from build123d import *

# Parameters (mm, degrees)
F0_R     = 2
F1_DEPTH = 12
F2_SIZE  = 2.286
F3_SIZE  = 2.286
F4_R     = 2.08915
F5_DEPTH = 219.3935


with BuildPart() as f1:
    # F0 (on Top) → F1 (new body)
    with BuildSketch(Plane.XY):
        with BuildLine():
            Line((12.08, 118.11), (5.08, 118.11))
            Line((5.08, 118.11), (5.08, 102.074511))
            Line((5.08, 102.074511), (0, 102.074511))
            Line((0, 102.074511), (19.539499, 37.638369))
            ThreePointArc((19.539499, 37.638369), (37.889981, 11.578561), (68.153533, 1.58))
            Line((68.153533, 1.58), (108.554348, 1.58))
            ThreePointArc((108.554348, 1.58), (107.15625, 5.08), (108.554348, 8.58))
            Line((108.554348, 8.58), (73.345626, 8.58))
            ThreePointArc((73.345626, 8.58), (43.082074, 18.578561), (24.731592, 44.638369))
            Line((24.731592, 44.638369), (15.358949, 75.546886))
            ThreePointArc((15.358949, 75.546886), (12.904195, 86.482216), (12.08, 97.659333))
            Line((12.08, 97.659333), (12.08, 118.11))
        make_face()
        with BuildLine():
            ThreePointArc((108.554348, 8.58), (107.15625, 5.08), (108.554348, 1.58))
            ThreePointArc((108.554348, 1.58), (112.23625, 0), (115.918152, 1.58))
            ThreePointArc((115.918152, 1.58), (116.953795, 3.195545), (117.31625, 5.08))
            ThreePointArc((117.31625, 5.08), (116.953795, 6.964455), (115.918152, 8.58))
            ThreePointArc((115.918152, 8.58), (112.23625, 10.16), (108.554348, 8.58))
        make_face()
        with Locations((112.23625, 5.08)):
            Circle(F0_R, mode=Mode.SUBTRACT)
        with BuildLine():
            ThreePointArc((117.31625, 5.08), (116.953795, 3.195545), (115.918152, 1.58))
            Line((115.918152, 1.58), (156.318967, 1.58))
            ThreePointArc((156.318967, 1.58), (186.582519, 11.578561), (204.933001, 37.638369))
            Line((204.933001, 37.638369), (224.4725, 102.074511))
            Line((224.4725, 102.074511), (219.3925, 102.074511))
            Line((219.3925, 102.074511), (219.3925, 118.11))
            Line((219.3925, 118.11), (212.3925, 118.11))
            Line((212.3925, 118.11), (212.3925, 97.659333))
            ThreePointArc((212.3925, 97.659333), (211.568305, 86.482216), (209.113551, 75.546886))
            Line((209.113551, 75.546886), (199.740908, 44.638369))
            ThreePointArc((199.740908, 44.638369), (181.390426, 18.578561), (151.126874, 8.58))
            Line((151.126874, 8.58), (115.918152, 8.58))
            ThreePointArc((115.918152, 8.58), (116.953795, 6.964455), (117.31625, 5.08))
        make_face()
    extrude(amount=-F1_DEPTH)

    # F2
    f2_edges = [f1.edges().sort_by_distance(p)[0] for p in [
        (110.23625, 5.08, 0),
    ]]
    chamfer(f2_edges, length=F2_SIZE)

    # F3
    f3_edges = [f1.edges().sort_by_distance(p)[0] for p in [
        (110.23625, 5.08, -12),
    ]]
    chamfer(f3_edges, length=F3_SIZE)

    # F4 (on face) → F5 (cut, through all)
    with BuildSketch(Plane(origin=(5.08, 0, 0), x_dir=(0, -1, 0), z_dir=(-1, 0, 0))):
        with Locations((-110.092256, -6)):
            Circle(F4_R)
    extrude(amount=-F5_DEPTH, mode=Mode.SUBTRACT)


solid = f1.part
Read the model definition and answer for the solid it produces. Units are mm, in the model's axes. A direction names the side the tool comes from. Give positions to 0.01 mm unless a question says otherwise; leave off trailing zeros. Write each loop counter-clockwise with the first axis right and the second up, starting at its lowest first coordinate (ties: lowest second). Pieces come first, ordered by that corner, then holes. Notation, with made-up numbers: (69, -23) - (84, -23) arc R22 cw to (84, 4) - close; hole circle Ø7 at (-25, 16). An arc over 180 degrees is marked (long way). Use CSV: the item, a comma, the result in double quotes. Start each with the question number.
(1) Given P1, Ø2.5, axis at y = 110.09, z = -6, coming from the -X side; P2, Ø1, axis at x = 155, z = -8.5, coming from the +Y side; P3, Ø3.5, axis at y = 109.5, z = -7.5, coming from the -X side; P4, Ø5, axis at y = 70.5, z = -9.5, coming from the -X side, each flat-ended and moving along its own axis, determine where each tip first touches the part or whether it passes through.
(2) Determine the mould class of faces 1 (the flat face through (216, 118.11, -6)), 2 (the flat face through (9.633, 70.307, -5.916)), 3 (the cylindrical face through (215.844, 108.162, -6.8)) for opening direction Y: +Y half, -Y half, draft (parallel to the pull), parting line (faces both ways), or undercut.
(3) Consider line 1 along X through (y, z) = (112.5, -6.5); line 2 along Y through (x, z) = (88.5, -6.75); line 3 along X through (y, z) = (19.5, -7.5). Determine where each line is inside the solid, lowest interval first.
(4) Find section C-C (x = 131.5). Give the vertices of the cut face in (y, z), plus the area to 3 significant figures.
(5) Find section A-A (z = -6). Count the separate pieces of the cut face and the enclosed holes in it, plus the area to 3 significant figures.
(6) Find section B-B (y = 78.5). Give the vertices of the cut face in (x, z).
(7) Find section D-D (y = 29). Give the vertices of the cut face in (x, z).
(8) For faces 4 (the flat face through (134, 8.58, -6)), 5 (the flat face through (88, 1.58, -6)), 6 (the flat face through (3, 102.075, -6)), 7 (the flat face through (222, 102.075, -6)), 8 (the conical face through (114.22, 4.26, -9.86)), determine the directions among +Z, -Z, +X, -X, +Y, -Y from which every point of the face is accessible in a straight line to the end or side of a thin tool.
Findings below:
1,P1,"through"
1,P2,"y = 8.77"
1,P3,"x = 5.08"
1,P4,"x = 8.82"
2,face 1,"+Y half"
2,face 2,"-Y half"
2,face 3,"undercut"
3,line 1,"5.08 to 12.08, 212.39 to 219.39"
3,line 2,"1.58 to 8.58"
3,line 3,"29.43 to 41.88, 182.59 to 195.04"
4,outline,"(1.58, -12) - (8.58, -12) - (8.58, 0) - (1.58, 0) - close"
4,area,"84.0 mm2"
5,separate pieces,"3"
5,enclosed holes,"1"
5,area,"2,780 mm2"
6,outline,"(7.15, -12) - (14.53, -12) - (14.53, 0) - (7.15, 0) - close; (209.94, -12) - (217.32, -12) - (217.32, 0) - (209.94, 0) - close"
7,outline,"(23.05, -12) - (32.63, -12) - (32.63, 0) - (23.05, 0) - close; (191.84, -12) - (201.42, -12) - (201.42, 0) - (191.84, 0) - close"
8,face 4,"+Z, -Z, +Y"
8,face 5,"+Z, -Z, -X, -Y"
8,face 6,"+Z, -Z, -X, +Y"
8,face 7,"+Z, -Z, +X, +Y"
8,face 8,"-Z"
